Could you check a few things on this drawing? It's one solid part, dimensions in mm from its lowest x, y, z. Round coordinates to 2 decimals unless told otherwise and drop trailing zeros. Write each loop counter-clockwise with the first axis right and the second up, starting at its lowest first coordinate (ties: lowest second). Pieces come first, ordered by that corner, then holes. Notation, with made-up numbers: (-13.75, 65.25) -> (32.25, 65.25) arc R15 cw to (32.25, 89.25) -> close; hole circle Ø4 at (29, -32.5). An arc over 180 degrees is marked (long way). Answer in a Markdown table with one row per item.
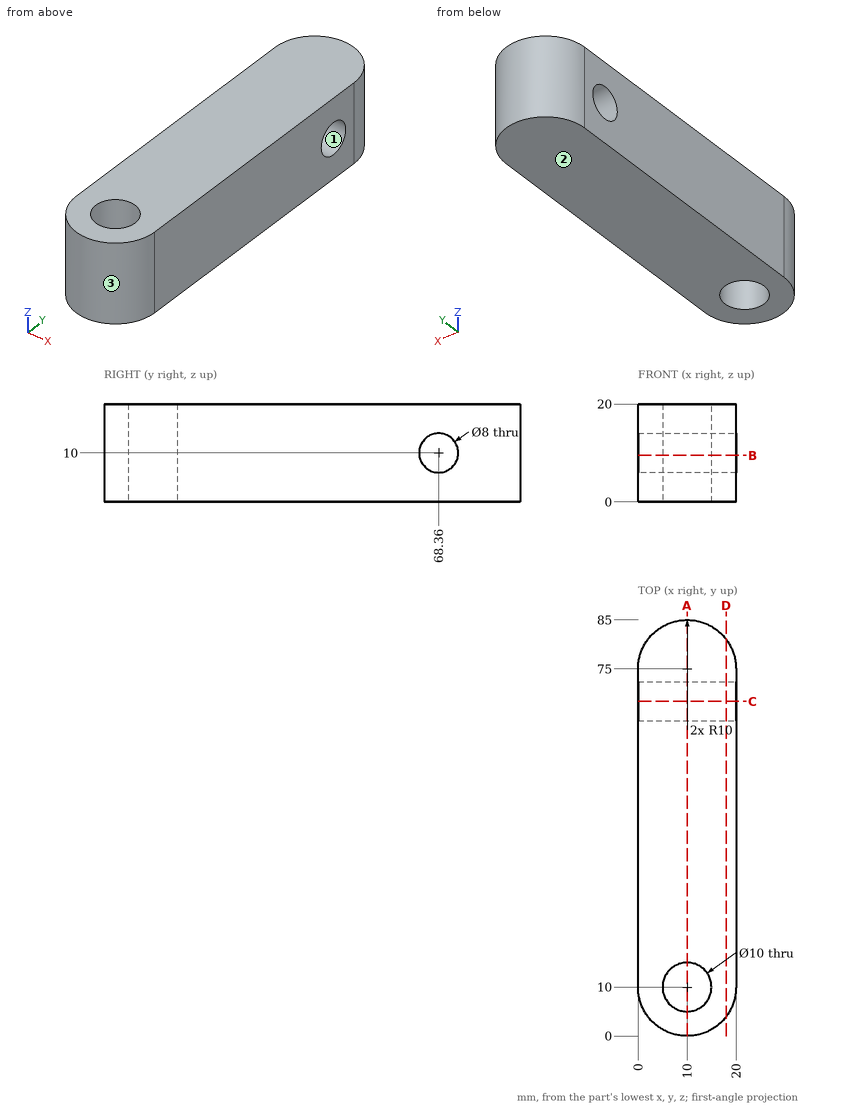
1) I want a section at A-A, the plane x = 10. List the corners of the cut face in (y, z) for me, and give its area (3 significant figures).
Response:
| item | result |
|---|---|
| outline | (0, 0) -> (5, 0) -> (5, 20) -> (0, 20) -> close; (15, 0) -> (85, 0) -> (85, 20) -> (15, 20) -> close; hole circle Ø8 at (68.36, 10) |
| area | 1,450 mm^2 |
2) For pin 1 (12 mm diameter, centred on x = 2, z = 6.5, fed in from -Y), with a flat end and sliding along its axis, tell me the tip position at first contact or that it passes through.
Response:
| item | result |
|---|---|
| pin 1 | stops at y = 0.2 |
3) I want a section at C-C, the plane y = 68.36. List the corners of the cut face in (x, z) for me, and give its area (3 significant figures).
Response:
| item | result |
|---|---|
| outline | (0, 0) -> (20, 0) -> (20, 6) -> (0, 6) -> close; (0, 14) -> (20, 14) -> (20, 20) -> (0, 20) -> close |
| area | 240 mm^2 |
4) I want a section at D-D, the plane x = 18. List the corners of the cut face in (y, z) for me, and give its area (3 significant figures).
Response:
| item | result |
|---|---|
| outline | (4, 0) -> (81, 0) -> (81, 20) -> (4, 20) -> close; hole circle Ø8 at (68.36, 10) |
| area | 1,490 mm^2 |
5) I need wall thicknesses on line 1 (Y direction, x = 12.25, z = 10); line 2 (Y direction, x = 14.5, z = 6.5); line 3 (Y direction, x = 10, z = 14.25). Which ranges of each line are inside material? Lowest first, please. Write a range as [from, to].
Response:
| item | result |
|---|---|
| line 1 | y = [0.26, 5.53], [14.47, 64.36], [72.36, 84.74] |
| line 2 | y = [1.07, 7.82], [12.18, 66.42], [70.3, 83.93] |
| line 3 | y = [0, 5], [15, 85] |
6) I want a section at B-B, the plane z = 9.5. List the corners of the cut face in (x, y) for me, and give its area (3 significant figures).
Response:
| item | result |
|---|---|
| outline | (0, 10) arc R10 ccw to (20, 10) -> (20, 64.39) -> (0, 64.39) -> close; (0, 72.33) -> (20, 72.33) -> (20, 75) arc R10 ccw to (0, 75) -> close; hole circle Ø10 at (10, 10) |
| area | 1,380 mm^2 |
7) We'd pull the mould along Y, two halves only. Please class the marked faces 1, 2 and 3: +Y half, -Y half, draft (parallel to the pull), parting line (faces both ways), or undercut.
Response:
| item | result |
|---|---|
| face 1 | undercut |
| face 2 | draft |
| face 3 | -Y half |
